from build123d import *

# Parameters (mm, degrees)
SKETCH_1_W          = 14
SKETCH_1_H          = 9
EXTRUDE_1_DEPTH     = 11
SKETCH_3_R          = 3
CUT_EXTRUDE_1_DEPTH = 8
SKETCH_5_R          = 0.6
EXTRUDE_2_DEPTH     = 7
CUT_EXTRUDE_2_DEPTH = 12
SKETCH_7_W          = 0.2
SKETCH_7_H          = 3
SKETCH_7_H_2        = 2.5
SKETCH_7_W_2        = 2.5
SKETCH_7_H_3        = 0.2
EXTRUDE_3_DEPTH     = 3


with BuildPart() as part:
    # 草图1 → 凸台-拉伸1 (new body)
    with BuildSketch(Plane.XY):
        Rectangle(SKETCH_1_W, SKETCH_1_H)
    extrude(amount=EXTRUDE_1_DEPTH)

    # 草图3 → 切除-拉伸1 (cut)
    with BuildSketch(Plane(origin=(7, 0, 0), x_dir=(0, 0, -1), z_dir=(1, 0, 0))):
        with Locations((-6, 0)):
            Circle(SKETCH_3_R)
    extrude(amount=-CUT_EXTRUDE_1_DEPTH, mode=Mode.SUBTRACT)

    # 草图5 → 凸台-拉伸2 (add)
    with BuildSketch(Plane(origin=(-1, 0, 0), x_dir=(0, 0, -1), z_dir=(1, 0, 0))):
        with Locations((-6, 0)):
            Circle(SKETCH_5_R)
    extrude(amount=EXTRUDE_2_DEPTH)

    # 草图6 → 切除-拉伸2 (cut)
    with BuildSketch(Plane.ZY.offset(7)):
        with BuildLine():
            Line((6, 4), (6, 4.5))
            Line((6, 4.5), (11, 4.5))
            Line((11, 4.5), (11, -4.5))
            Line((11, -4.5), (6, -4.5))
            Line((6, -4.5), (6, -4))
            ThreePointArc((6, -4), (10, 0), (6, 4))
        make_face()
    extrude(amount=-CUT_EXTRUDE_2_DEPTH, mode=Mode.SUBTRACT)

    # 草图7 → 凸台-拉伸3 (add)
    with BuildSketch(Plane(origin=(0, 0, 0), x_dir=(-1, 0, 0), z_dir=(0, 0, -1))):
        with Locations((6.9, 0)):
            Rectangle(SKETCH_7_W, SKETCH_7_H)
        with Locations((-0.1, 0)):
            Rectangle(SKETCH_7_W, SKETCH_7_H_2)
        with Locations((3.9, 4.4)):
            Rectangle(SKETCH_7_W_2, SKETCH_7_H_3)
    extrude(amount=EXTRUDE_3_DEPTH)


solid = part.part
Geometry: final body of the model. Coordinates: model frame, mm. A direction names the side the tool comes from. Round coordinates to 2 decimals unless told otherwise and drop trailing zeros. Loops run counter-clockwise (first coordinate to the right, second up) from the corner with the lowest first, then second, coordinate; pieces in that order, holes last.
Q1. Section B-B on z = -1. Return loops of the section in (x, y).
Q2. Pull-direction query (Z, two-part tool) for faces 1 (the flat face through (6, 0, 11)), 2 (the flat face through (6, 0, 6)), 3 (the flat face through (0, -4.5, 3)); classes: released by +Z, released by -Z, zero draft, split by the parting line, or undercut.
Q3. Section D-D on y = 0. Return loops of the section in (x, z).
Q4. Section C-C on x = -3.25. Return loops of the section in (y, z).
Q5. Material intervals for L1, parallel to X at y = 0.5, z = -2.25; L2, parallel to X at y = -1.75, z = 4.75; L3, parallel to X at y = 4.25, z = 6.5, sorted ascending.
Q6. Section A-A on x = 3. Return loops of the section in (y, z).
Q7. Pin query (flat end, axial travel): P1, Ø1, axis at y = 0, z = 6, coming from the +X side; P2, Ø1, axis at x = 3, z = 9, coming from the -Y side; P3, Ø1.5, axis at x = 3, y = -3.5, coming from the +Z side. Return the tip coordinate at first contact, or that it passes through.
Q8. Access query for faces 4 (the flat face through (0.2, 0, -1)), 5 (the flat face through (5, 0.1, 10.2)), 6 (the cylindrical face through (2.451, 0.18, 5.428)), 7 (the flat face through (0, 0, -1)), 8 (the flat face through (-4, 4.3, -1)). Directions: +Z, -Z, +X, -X, +Y, -Y. A direction counts if a zero-diameter tool reaches every point of the face in a straight line with its end or side. Return the directions, or none.
Evaluation:
1. outline: (-7, -1.5) - (-6.8, -1.5) - (-6.8, 1.5) - (-7, 1.5) - close; (-5.15, 4.3) - (-2.65, 4.3) - (-2.65, 4.5) - (-5.15, 4.5) - close; (0, -1.25) - (0.2, -1.25) - (0.2, 1.25) - (0, 1.25) - close
2. face 1: released by +Z
2. face 2: undercut
2. face 3: zero draft
3. outline: (-7, -3) - (-6.8, -3) - (-6.8, 0) - (0, 0) - (0, -3) - (0.2, -3) - (0.2, 0) - (7, 0) - (7, 3) - (-1, 3) - (-1, 5.4) - (6, 5.4) - (6, 6.6) - (-1, 6.6) - (-1, 9) - (7, 9) - (7, 11) - (5, 11) - (5, 10) - (-7, 10) - close
4. outline: (-4.5, 0) - (4.3, 0) - (4.3, -3) - (4.5, -3) - (4.5, 6) - (4, 6) arc R4 ccw to (-4, 6) - (-4.5, 6) - close
5. L1: x = -7 to -6.8, 0 to 0.2
5. L2: x = -7 to -1
5. L3: x = 5 to 7
6. outline: (-4.5, 0) - (4.5, 0) - (4.5, 6) - (4, 6) arc R4 ccw to (-4, 6) - (-4.5, 6) - close; circle Ø1.2 at (0, 6); hole circle Ø6 at (0, 6)
7. P1: stops at x = 6
7. P2: stops at y = -3.12
7. P3: stops at z = 8.9
8. face 4: -Z, +X, +Y, -Y
8. face 5: +Z, -X
8. face 6: +X
8. face 7: -Z, +Y, -Y
8. face 8: -Z, +X, -X, -Y
